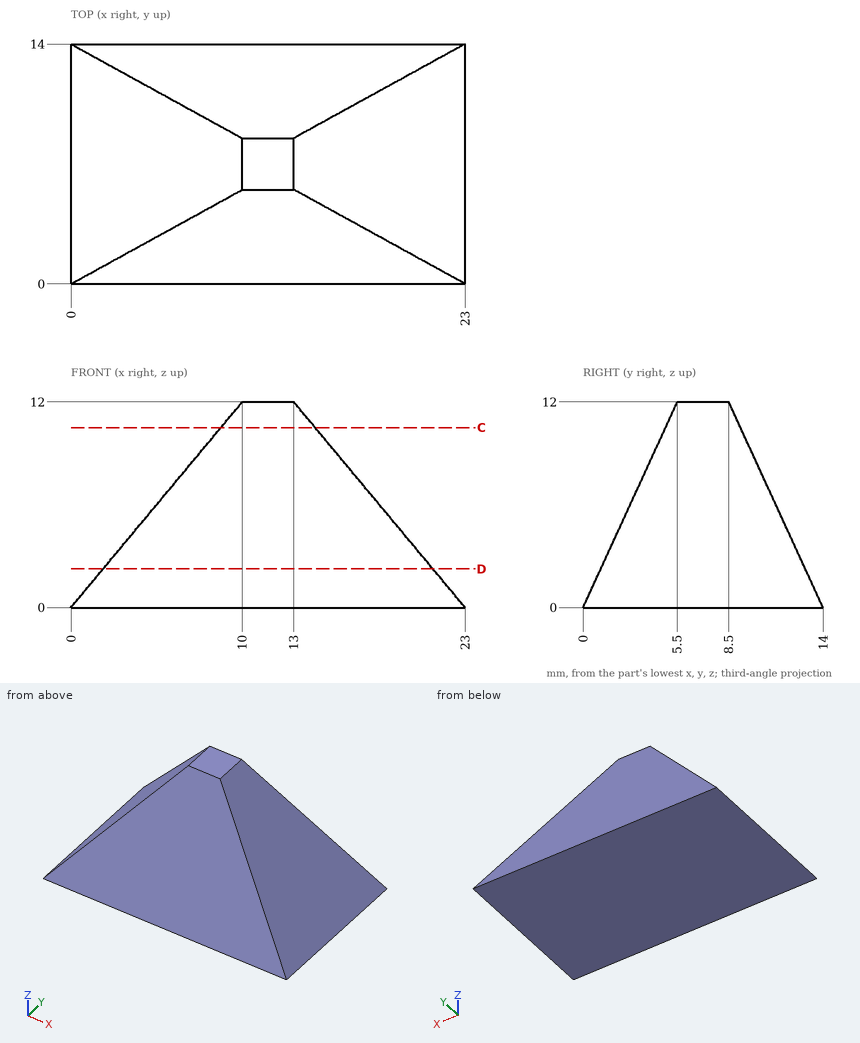
Print and shaded views of the part. All mm, measured from the part's lowest x, y and z. Give positions to 0.01 mm unless a question says otherwise; leave off trailing zeros. Loops run counter-clockwise (first coordinate to the right, second up) from the corner with the lowest first, then second, coordinate; pieces in that order, holes last. Notation, with made-up numbers: (32, 60) -> (48, 60) arc R25 cw to (48, 77) -> close; hole circle Ø6 at (2.5, -21). An arc over 180 degrees is marked (long way). One line per question, with ' | ' between items. Start each with the question number.
1) Cut at C-C (z = 10.5). Give the cut face in (x, y).
2) Cut at D-D (z = 2.25). Give the cut face in (x, y) (3 decimals), plus the area to 3 significant figures.
3) Pin check, flat tips, straight feed: pin 1 (2 mm diameter, centred on x = 2.5, z = 3.5, fed in from -Y); pin 2 (6 mm diameter, centred on y = 3, z = 9.5, fed in from +X); pin 3 (3 mm diameter, centred on x = 11, y = 12, fed in from +Z). Stop position of each tip, or through.
4) Probe L1, parallel to Z at x = 15.5, y = 3.5; L2, parallel to Z at x = 19.25, y = 1.5; L3, parallel to Y at x = 4, z = 1. List the from-to ranges inside material, lowest first.
Return value:
1) outline: (8.75, 4.81) -> (14.25, 4.81) -> (14.25, 9.19) -> (8.75, 9.19) -> close
2) outline: (1.875, 1.031) -> (21.125, 1.031) -> (21.125, 12.969) -> (1.875, 12.969) -> close | area: 230 mm^2
3) pin 1: y = 1.15 | pin 2: x = 17.58 | pin 3: z = 7.64
4) L1: 0 to 7.64 | L2: 0 to 3.27 | L3: 0.46 to 13.54
